```python
from build123d import *

# Parameters (mm, degrees)
SKETCH1_W           = 27.3
SKETCH1_H           = 25.5
BOSS_EXTRUDE1_DEPTH = 10
CUT_EXTRUDE1_DEPTH  = 0.9
SKETCH3_R           = 7.8
BOSS_EXTRUDE2_DEPTH = 9.4
SKETCH4_R           = 5.95
BOSS_EXTRUDE3_DEPTH = 3.8
SKETCH5_R           = 7
BOSS_EXTRUDE4_DEPTH = 4.3
SKETCH6_R           = 5.25
CUT_EXTRUDE2_DEPTH  = 0.5
SKETCH7_W           = 6.9
SKETCH7_H           = 3.2
BOSS_EXTRUDE5_DEPTH = 1.1
SKETCH8_W           = 5.9
SKETCH8_H           = 2.7
CUT_EXTRUDE3_DEPTH  = 2.5


with BuildPart() as part:
    # Sketch1 → Boss-Extrude1 (new body)
    with BuildSketch(Plane(origin=(0, 0, 0), x_dir=(1, 0, 0), z_dir=(0, 1, 0))):
        Rectangle(SKETCH1_W, SKETCH1_H)
    extrude(amount=BOSS_EXTRUDE1_DEPTH)

    # Sketch2 → Cut-Extrude1 (cut)
    with BuildSketch(Plane(origin=(0, 10, 0), x_dir=(1, 0, 0), z_dir=(0, 1, 0))):
        with BuildLine():
            Line((-8.2, 5.981847541), (-8.2, 12.75))
            Line((-8.2, 12.75), (-13.65, 12.75))
            Line((-13.65, 12.75), (-13.65, -12.75))
            Line((-13.65, -12.75), (-8.2, -12.75))
            Line((-8.2, -12.75), (-8.2, -5.981847541))
            ThreePointArc((-8.2, -5.981847541), (-10.15, 0), (-8.2, 5.981847541))
        make_face()
        with BuildLine():
            Line((13.65, 12.75), (8.2, 12.75))
            Line((8.2, 12.75), (8.2, 5.981847541))
            ThreePointArc((8.2, 5.981847541), (9.650194299, 3.145830574), (10.15, 0))
            ThreePointArc((10.15, 0), (9.650194299, -3.145830574), (8.2, -5.981847541))
            Line((8.2, -5.981847541), (8.2, -12.75))
            Line((8.2, -12.75), (13.65, -12.75))
            Line((13.65, -12.75), (13.65, 12.75))
        make_face()
        with BuildLine():
            ThreePointArc((0, -10.15), (-2.310672611, -9.883485827), (-4.5, -9.097939327))
            Line((-4.5, -9.097939327), (-4.5, -12.75))
            Line((-4.5, -12.75), (0, -12.75))
            Line((0, -12.75), (0, -10.15))
        make_face()
        with BuildLine():
            ThreePointArc((4.5, -9.097939327), (2.310672611, -9.883485827), (0, -10.15))
            Line((0, -10.15), (0, -12.75))
            Line((0, -12.75), (4.5, -12.75))
            Line((4.5, -12.75), (4.5, -9.097939327))
        make_face()
    extrude(amount=-CUT_EXTRUDE1_DEPTH, mode=Mode.SUBTRACT)

    # Sketch3 → Boss-Extrude2 (add)
    with BuildSketch(Plane(origin=(0, 10, 0), x_dir=(1, 0, 0), z_dir=(0, 1, 0))):
        with Locations(Location((0, 0, 0), (0, 0, 270))):
            Circle(SKETCH3_R)
    extrude(amount=BOSS_EXTRUDE2_DEPTH)

    # Sketch4 → Boss-Extrude3 (add)
    with BuildSketch(Plane(origin=(0, 19.4, 0), x_dir=(1, 0, 0), z_dir=(0, 1, 0))):
        with Locations(Location((0, 0, 0), (0, 0, 90))):
            Circle(SKETCH4_R)
    extrude(amount=BOSS_EXTRUDE3_DEPTH)

    # Sketch5 → Boss-Extrude4 (add)
    with BuildSketch(Plane(origin=(0, 23.2, 0), x_dir=(1, 0, 0), z_dir=(0, 1, 0))):
        with Locations(Location((0, 0, 0), (0, 0, 270))):
            Circle(SKETCH5_R)
    extrude(amount=BOSS_EXTRUDE4_DEPTH)

    # Sketch6 → Cut-Extrude2 (cut)
    with BuildSketch(Plane(origin=(0, 27.5, 0), x_dir=(1, 0, 0), z_dir=(0, 1, 0))):
        with Locations(Location((0, 0, 0), (0, 0, 270))):
            Circle(SKETCH6_R)
    extrude(amount=-CUT_EXTRUDE2_DEPTH, mode=Mode.SUBTRACT)

    # Sketch7 → Boss-Extrude5 (add)
    with BuildSketch(Plane.XZ):
        with Locations((0, 9.65)):
            Rectangle(SKETCH7_W, SKETCH7_H)
    extrude(amount=BOSS_EXTRUDE5_DEPTH)

    # Sketch8 → Cut-Extrude3 (cut)
    with BuildSketch(Plane.XZ.offset(1.1)):
        with Locations((0, 9.4)):
            Rectangle(SKETCH8_W, SKETCH8_H)
    extrude(amount=-CUT_EXTRUDE3_DEPTH, mode=Mode.SUBTRACT)


solid = part.part
```
Geometry check sheet. Reference: the model listing, model coordinates, mm. A direction names the side the tool comes from. Coordinates: 2 decimals unless noted, no trailing zeros. Order: outer loops, then holes, each group sorted by start corner. A loop starts at its lowest first (then second) coordinate and runs counter-clockwise, first axis right, second up. Notation, with made-up numbers: (69, -11) - (86, -11) arc R25 ccw to (86, 2) - close; hole circle Ø1 at (22.25, 55.25). An arc over 180 degrees is marked (long way). Answer as a JSON object with one key per item and string values. Group by question number.
Item 1: Sectioned sample at A-A, the plane y = 24.25. Record the cut outline in (x, z).
Item 2: Scan lines: probe 1 along X at (y, z) = (27.1, 0); probe 2 along Y at (x, z) = (1.5, 1.5); probe 3 along Y at (x, z) = (-6, 7.5). Record each from-to range of solid material in increasing order.
Item 3: Sectioned sample at D-D, the plane y = 17.5. Record the cut outline in (x, z), and give its area (3 significant figures).
Item 4: Tool access check on faces 1 (the face through (-6, 23.2, -2)), 2 (the face through (3.45, -0.5, 9.6)), 3 (the face through (-11, 9.1, 0)). Record the directions out of +Z, -Z, +X, -X, +Y, -Y that give a thin tool (end or side, any length) a straight path to the whole face; none if there is none.
Item 5: Sectioned sample at C-C, the plane x = -11.25. Record the cut outline in (y, z).
Item 6: Depth check by flat-ended pin: pin 1 Ø0.9 at (x, y) = (1, -0.5) entering from +Z; pin 2 Ø1.3 at (x, z) = (1.5, 10) entering from -Y; pin 3 Ø10 at (x, z) = (4, -2) entering from +Y; pin 4 Ø1.6 at (x, z) = (12, -1) entering from +Y. Enter the tip coordinate at first touch or a pass-through.
Item 7: Sectioned sample at B-B, the plane z = 3.5. Record the cut outline in (x, y).
Item 8: Draft check along X on faces 4 (the face through (-6.834, 25.32, -1.517)), 5 (the face through (-4.5, 9.6, 10.9)), 6 (the face through (4.5, 9.6, 10.9)), 7 (the face through (-3.45, -0.5, 9.6)). Enter one of: +X half, -X half, draft (parallel to the pull), parting line (faces both ways), or undercut.
Resolved:
{
 "1": {"outline": "circle Ø14 at (0, 0)"},
 "2": {"probe 1": "-7 to -5.25, 5.25 to 7", "probe 2": "0 to 27", "probe 3": "0 to 10"},
 "3": {"outline": "circle Ø15.6 at (0, 0)", "area": "191 mm^2"},
 "4": {"face 1": "none", "face 2": "+Z, -Z, +X, -Y", "face 3": "-X, +Y"},
 "5": {"outline": "(0, -12.75) - (9.1, -12.75) - (9.1, 12.75) - (0, 12.75) - close"},
 "6": {"pin 1": "z = 11.25", "pin 2": "y = 1.4", "pin 3": "y = 27.5", "pin 4": "y = 9.1"},
 "7": {"outline": "(-13.65, 0) - (13.65, 0) - (13.65, 9.1) - (9.53, 9.1) - (9.53, 10) - (6.97, 10) - (6.97, 19.4) - (4.81, 19.4) - (4.81, 23.2) - (6.06, 23.2) - (6.06, 27.5) - (3.91, 27.5) - (3.91, 27) - (-3.91, 27) - (-3.91, 27.5) - (-6.06, 27.5) - (-6.06, 23.2) - (-4.81, 23.2) - (-4.81, 19.4) - (-6.97, 19.4) - (-6.97, 10) - (-9.53, 10) - (-9.53, 9.1) - (-13.65, 9.1) - close"},
 "8": {"face 4": "parting line", "face 5": "undercut", "face 6": "undercut", "face 7": "-X half"}
}
